Model file for the job. Use its own axes, mm. A direction names the side the tool comes from. Round coordinates to 2 decimals unless told otherwise and drop trailing zeros. Loops run counter-clockwise (first coordinate to the right, second up) from the corner with the lowest first, then second, coordinate; pieces in that order, holes last. Notation, with made-up numbers: M 42,65 L 101,65 A10 cw 101,84 Z; hole C 86,-9.5 d1. An arc over 180 degrees is marked long. Answer in a Markdown table with one row per item.
from build123d import *

# Parameters (mm, degrees)
F0_W      = 114.808
F0_H      = 63.5
F1_DEPTH  = 6.35
F2_W      = 6.35
F2_H      = 63.5
F3_DEPTH  = 21.082
F4_W      = 121.158
F4_H      = 6.35
F5_DEPTH  = 21.082
F6_W      = 6.35
F6_H      = 69.85
F7_DEPTH  = 21.082
F8_W      = 6.35
F8_H      = 63.5
F9_DEPTH  = 3.81
F10_W     = 108.458
F10_H     = 6.35
F11_DEPTH = 3.81
F12_W     = 6.35
F12_H     = 57.15
F13_DEPTH = 3.81
F14_W     = 50.0406362116
F14_H     = 73.5886525363
F15_DEPTH = 6.35
F17_D     = 6.35


with BuildPart() as f1:
    # F0 (on Top) → F1 (new body)
    with BuildSketch(Plane.XY):
        Rectangle(F0_W, F0_H)
    extrude(amount=F1_DEPTH)

    # F2 (on Top) → F3 (join)
    with BuildSketch(Plane.XY):
        with Locations((-60.579, 0)):
            Rectangle(F2_W, F2_H)
    extrude(amount=F3_DEPTH)

    # F4 (on Top) → F5 (join)
    with BuildSketch(Plane.XY):
        with Locations((-3.175, -34.925)):
            Rectangle(F4_W, F4_H)
    extrude(amount=F5_DEPTH)

    # F6 (on Top) → F7 (join)
    with BuildSketch(Plane.XY):
        with Locations((60.579, -3.175)):
            Rectangle(F6_W, F6_H)
    extrude(amount=F7_DEPTH)

    # F8 (on face) → F9 (join)
    with BuildSketch(Plane.XY.offset(21.082)):
        with Locations((54.229, 0)):
            Rectangle(F8_W, F8_H)
        Polygon((63.754, -38.1), (63.754, 31.75), (57.404, 31.75), (57.404, -31.75), (51.054, -31.75), (51.054, -38.1), align=None)
    extrude(amount=F9_DEPTH)

    # F10 (on face) → F11 (join)
    with BuildSketch(Plane.XY.offset(21.082)):
        Polygon((-63.754, -25.4), (-63.754, -38.1), (51.054, -38.1), (51.054, -31.75), (-57.404, -31.75), (-57.404, -25.4), align=None)
        with Locations((-3.175, -28.575)):
            Rectangle(F10_W, F10_H)
    extrude(amount=F11_DEPTH)

    # F12 (on face) → F13 (join)
    with BuildSketch(Plane.XY.offset(21.082)):
        with Locations((-60.579, 3.175)):
            Rectangle(F12_W, F12_H)
        with Locations((-54.229, 3.175)):
            Rectangle(F12_W, F12_H)
    extrude(amount=F13_DEPTH)

    # F14 (on Top) → F15 (join)
    with BuildSketch(Plane.XY):
        with Locations((0, 31.7919999361)):
            Rectangle(F14_W, F14_H)
    extrude(amount=F15_DEPTH)

    # F17 (through all)
    with Locations(Plane.XY.offset(6.35)):
        with Locations((0, 50.6303012371)):
            Hole(F17_D / 2)


solid = f1.part
1. Saw through at D-D (z = 11.5). Write the cut outline in (x, y), and give its area (3 significant figures).
Verdict:
| item | result |
|---|---|
| outline | M -63.75,-38.1 L 63.75,-38.1 L 63.75,31.75 L 57.4,31.75 L 57.4,-31.75 L -57.4,-31.75 L -57.4,31.75 L -63.75,31.75 Z |
| area | 1,620 mm² |
2. Tool access for faces 1 (the flat face through (-9, -26, 21.082)), 2 (the flat face through (-50, 31.75, 6)), 3 (the flat face through (53, 31.75, 4)), 4 (the flat face through (-51.054, 3, 23)): list every direction of +Z, -Z, +X, -X, +Y, -Y with a clear straight run to the whole face (end or side of a thin tool).
Verdict:
| item | result |
|---|---|
| face 1 | +Y |
| face 2 | +Z, -Z, -X, +Y |
| face 3 | +Z, -Z, +X, +Y |
| face 4 | +Z, +Y |
3. Pin check, flat tips, straight feed: pin 1 (3 mm diameter, centred on x = 13.5, z = 22.5, fed in from +Y); pin 2 (3 mm diameter, centred on y = 56.5, z = 4, fed in from +X); pin 3 (5.5 mm diameter, centred on x = 0, y = 50.63, fed in from -Z); pin 4 (1 mm diameter, centred on x = 33.5, z = 13.5, fed in from +Y). Stop position of each tip, or through.
Verdict:
| item | result |
|---|---|
| pin 1 | stops at y = -25.4 |
| pin 2 | stops at x = 25.02 |
| pin 3 | passes through |
| pin 4 | stops at y = -31.75 |
4. Saw through at B-B (y = 16). Write the cut outline in (x, z), and give its area (3 significant figures).
Verdict:
| item | result |
|---|---|
| outline | M -63.75,0 L 63.75,0 L 63.75,24.89 L 51.05,24.89 L 51.05,21.08 L 57.4,21.08 L 57.4,6.35 L -57.4,6.35 L -57.4,21.08 L -51.05,21.08 L -51.05,24.89 L -63.75,24.89 Z |
| area | 1,090 mm² |
5. Saw through at A-A (x = 0). Write the cut outline in (y, z), and give its area (3 significant figures).
Verdict:
| item | result |
|---|---|
| outline | M -38.1,0 L 47.46,0 L 47.46,6.35 L -31.75,6.35 L -31.75,21.08 L -25.4,21.08 L -25.4,24.89 L -38.1,24.89 Z; M 53.81,0 L 68.59,0 L 68.59,6.35 L 53.81,6.35 Z |
| area | 779 mm² |
6. Saw through at C-C (x = -32.5). Write the cut outline in (y, z).
Verdict:
| item | result |
|---|---|
| outline | M -38.1,0 L 31.75,0 L 31.75,6.35 L -31.75,6.35 L -31.75,21.08 L -25.4,21.08 L -25.4,24.89 L -38.1,24.89 Z |
7. Mould opens along Z. For faces 5 (the flat face through (0, 68.586, 3)), 6 (the flat face through (-1, -26, 24.892)), 7 (the flat face through (-1, -31.75, 14)), 8 (the flat face through (57.404, 0, 14)) say: +Z half, -Z half, draft (parallel to the pull), parting line (faces both ways), or undercut.
Verdict:
| item | result |
|---|---|
| face 5 | draft |
| face 6 | +Z half |
| face 7 | undercut |
| face 8 | undercut |
8. Wall check: probe 1 along Y at (x, z) = (0, 4.75); probe 2 along X at (y, z) = (-11, 11.25); probe 3 along Z at (x, y) = (2, -28.5). Give the ranges that are in metal, low to high.
Verdict:
| item | result |
|---|---|
| probe 1 | y = -38.1 to 47.46, 53.81 to 68.59 |
| probe 2 | x = -63.75 to -57.4, 57.4 to 63.75 |
| probe 3 | z = 0 to 6.35, 21.08 to 24.89 |
